The model under review builds one solid part; all positions refer to its coordinate system, in mm. Face numbers are marked on the shaded views. Round coordinates to 2 decimals unless told otherwise and drop trailing zeros. Order: outer loops, then holes, each group sorted by start corner. A loop starts at its lowest first (then second) coordinate and runs counter-clockwise, first axis right, second up. Notation, with made-up numbers: (30, 7) -> (88, 7) arc R9 cw to (88, 20) -> close; hole circle Ø8 at (25, 3.5). An arc over 180 degrees is marked (long way). Put each result on its own line as item: value. Start each with the question number.
from build123d import *

# Parameters (mm, degrees)
SKETCH1_W             = 30
SKETCH1_H             = 15
BOSS_EXTRUDE1_DEPTH   = 15
FILLET1_R             = 2.5
M5_TAPPED_HOLE1_D     = 4.2
M5_TAPPED_HOLE1_DEPTH = 12.4
M5_TAPPED_HOLE1_TIP   = 1.2618073
M2_TAPPED_HOLE1_D     = 1.6
M2_TAPPED_HOLE1_DEPTH = 5
M2_TAPPED_HOLE1_TIP   = 0.480688495


with BuildPart() as part:
    # Sketch1 → Boss-Extrude1 (new body)
    with BuildSketch(Plane(origin=(0, 0, 0), x_dir=(1, 0, 0), z_dir=(0, 1, 0))):
        Rectangle(SKETCH1_W, SKETCH1_H)
    extrude(amount=BOSS_EXTRUDE1_DEPTH)

    # Fillet1
    fillet1_edges = [part.edges().sort_by_distance(p)[0] for p in [
        (-15, 7.5, -7.5),
        (15, 7.5, -7.5),
    ]]
    fillet(fillet1_edges, radius=FILLET1_R)

    # M5 Tapped Hole1
    with Locations(Plane(origin=(0, 15, 0), x_dir=(1, 0, 0), z_dir=(0, 1, 0))):
        with Locations((-7.5, 1.25), (7.5, 1.25)):
            Hole(M5_TAPPED_HOLE1_D / 2, depth=M5_TAPPED_HOLE1_DEPTH)
            with Locations((0, 0, -(M5_TAPPED_HOLE1_DEPTH + M5_TAPPED_HOLE1_TIP / 2))):  # 118° drill point
                Cone(0, M5_TAPPED_HOLE1_D / 2, M5_TAPPED_HOLE1_TIP, mode=Mode.SUBTRACT)

    # M2 Tapped Hole1
    with Locations(Plane.XY.offset(7.5)):
        with Locations((7.5, 7.5), (-7.5, 7.5)):
            Hole(M2_TAPPED_HOLE1_D / 2, depth=M2_TAPPED_HOLE1_DEPTH)
            with Locations((0, 0, -(M2_TAPPED_HOLE1_DEPTH + M2_TAPPED_HOLE1_TIP / 2))):  # 118° drill point
                Cone(0, M2_TAPPED_HOLE1_D / 2, M2_TAPPED_HOLE1_TIP, mode=Mode.SUBTRACT)


solid = part.part
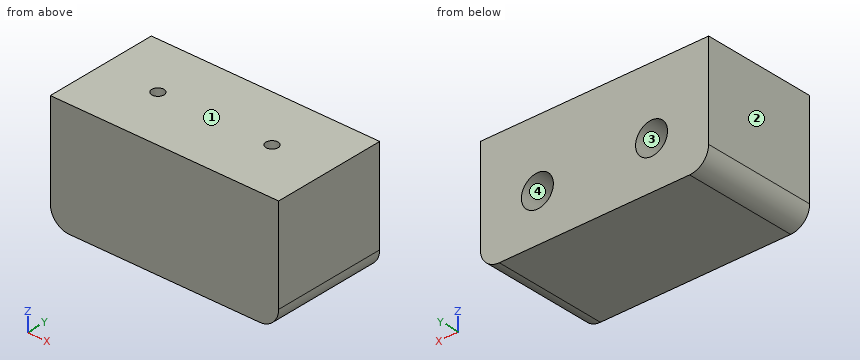
Q1. Take a section at A-A on y = 9. Give the boundary of the cut face in (x, z), and give its area (3 significant figures).
Q2. Clearance check with a flat-ended pin moving along its axis: pin 1 Ø1 at (x, y) = (-7.5, 7.5) entering from +Z. State where the tip first meets the part, or that it passes through.
Q3. Wall thickness on probe 1 along X at (y, z) = (7.5, 5.1); probe 2 along Z at (x, y) = (7.5, 9); probe 3 along Y at (x, z) = (7.5, 3): over which ranges is each line inside the solid? List them lowest first. Write a range as [from, to].
Q4. Draft analysis for pull direction Z (two halves, no side actions). For the marked faces 1, 2, 3 and 4, state which applies: +Z half, -Z half, draft (parallel to the pull), parting line (faces both ways), or undercut.
Calculated:
1. outline: (-15, -5) arc R2.5 ccw to (-12.5, -7.5) -> (12.5, -7.5) arc R2.5 ccw to (15, -5) -> (15, 7.5) -> (-15, 7.5) -> close; hole circle Ø4.2 at (-7.5, -1.25); hole circle Ø4.2 at (7.5, -1.25)
1. area: 420 mm²
2. pin 1: stops at z = 2.32
3. probe 1: x = [-15, -8.3], [-6.7, 6.7], [8.3, 15]
3. probe 2: z = [-7.5, -3.35], [0.85, 7.5]
3. probe 3: y = [0, 6.7], [8.3, 15]
4. face 1: +Z half
4. face 2: draft
4. face 3: undercut
4. face 4: undercut
